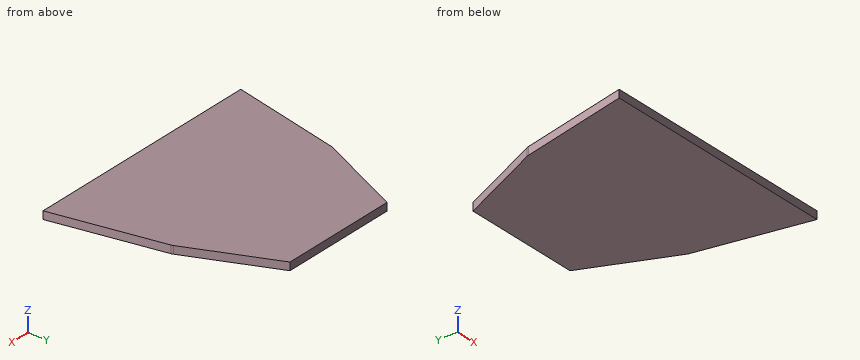
Autodesk Inventor part; units mm, degrees
ref_plane "Work Plane1" through (16.5341, 952.9567, 0) normal (0, 0, 1) x (-1, 0, 0)
ref_plane "YZ Plane" through (0, 0, 0) normal (1, 0, 0) x (0, 1, 0)
ref_plane "XZ Plane" through (0, 0, 0) normal (0, 1, 0) x (-1, 0, 0)
ref_plane "Work Plane1" through (16.5341, 952.9567, 0) normal (0, 0, 1) x (-1, 0, 0)
sketch "Sketch1" plane through (16.5341, 952.9567, 0) normal (0, 0, 1) x (-1, 0, 0)
  line L0 (60, 40.2719) -> (60, 137.1193)
  ellipse E0 centre (56, 137.1193) end of major axis (56, 141.9614) minor radius 4 (60, 137.1193) -> (56, 141.9614) ccw
  line L1 (56, 141.9614) -> (24.75, 141.9614)
  line L2 (24.75, 141.9614) -> (24.75, 144.3824)
  line L3 (24.75, 144.3824) -> (24.75, 146.8034)
  line L4 (24.75, 146.8034) -> (56, 146.8034)
  ellipse E1 centre (56, 137.1193) end of major axis (56, 146.8034) minor radius 8 (64, 137.1193) -> (56, 146.8034) ccw
  line L5 (64, 137.1193) -> (64, 40.2719)
  ellipse E2 centre (56, 40.2719) end of major axis (56, 30.5879) minor radius 8 (63.7591, 37.9134) -> (64, 40.2719) ccw
  line L6 (63.7591, 37.9134) -> (43.4204, -60.1335)
  ellipse E3 centre (35.6613, -57.775) end of major axis (35.6613, -67.459) minor radius 8 (42.7123, -62.3499) -> (43.4204, -60.1335) ccw
  line L7 (42.7123, -62.3499) -> (7.051, -142.8866)
  ellipse E4 centre (0, -138.3116) end of major axis (0, -147.9957) minor radius 8 (-7.051, -142.8866) -> (7.051, -142.8866) ccw
  line L8 (-7.051, -142.8866) -> (-42.7123, -62.3499)
  ellipse E5 centre (-35.6613, -57.775) end of major axis (-35.6613, -67.459) minor radius 8 (-43.4204, -60.1335) -> (-42.7123, -62.3499) ccw
  line L9 (-43.4204, -60.1335) -> (-63.7591, 37.9134)
  ellipse E6 centre (-56, 40.2719) end of major axis (-56, 30.5879) minor radius 8 (-64, 40.2719) -> (-63.7591, 37.9134) ccw
  line L10 (-64, 40.2719) -> (-64, 137.1193)
  ellipse E7 centre (-56, 137.1193) end of major axis (-56, 146.8034) minor radius 8 (-56, 146.8034) -> (-64, 137.1193) ccw
  line L11 (-56, 146.8034) -> (-24.75, 146.8034)
  line L12 (-24.75, 146.8034) -> (-24.75, 144.3824)
  line L13 (-24.75, 144.3824) -> (-24.75, 141.9614)
  line L14 (-24.75, 141.9614) -> (-56, 141.9614)
  ellipse E8 centre (-56, 137.1193) end of major axis (-56, 141.9614) minor radius 4 (-56, 141.9614) -> (-60, 137.1193) ccw
  line L15 (-60, 137.1193) -> (-60, 40.2719)
  ellipse E9 centre (-56, 40.2719) end of major axis (-56, 35.4299) minor radius 4 (-60, 40.2719) -> (-59.8796, 39.0927) ccw
  line L16 (-59.8796, 39.0927) -> (-39.5409, -58.9542)
  ellipse E10 centre (-35.6613, -57.775) end of major axis (-35.6613, -62.617) minor radius 4 (-39.5409, -58.9542) -> (-39.1868, -60.0624) ccw
  line L17 (-39.1868, -60.0624) -> (-3.5255, -140.5991)
  ellipse E11 centre (0, -138.3116) end of major axis (0, -143.1536) minor radius 4 (-3.5255, -140.5991) -> (3.5255, -140.5991) ccw
  line L18 (3.5255, -140.5991) -> (39.1868, -60.0624)
  ellipse E12 centre (35.6613, -57.775) end of major axis (35.6613, -62.617) minor radius 4 (39.1868, -60.0624) -> (39.5409, -58.9542) ccw
  line L19 (39.5409, -58.9542) -> (59.8796, 39.0927)
  ellipse E13 centre (56, 40.2719) end of major axis (56, 35.4299) minor radius 4 (59.8796, 39.0927) -> (60, 40.2719) ccw
  line L20 (-24.75, 141.9614) -> (24.75, 141.9614)
  line L21 (-24.0389, -94.2722) -> (24.0389, -94.2722)
  line L22 (-48.8096, -14.2722) -> (48.8096, -14.2722)
  point P0 (16.5341, 952.9567)
  point P1 (60, -19.5271)
  dimension "d3" = 88.0788
  dimension "d4" = 44.0394
  dimension "d12" = 80
extrude "Plate1" add sketch "Sketch1" along normal blind 3 contours L19 E12 L18 L21 L17 E10 L16 L22
ref_plane "modplan parallel med plade" through (16.5341, 952.9567, 1.5) normal (0, 0, 1) x (1, 0, 0)
sketch "Sketch3" plane through (16.5341, 952.9567, 0) normal (0, 0, -1) x (-1, 0, 0)
  ellipse E0 centre (-35.6613, 57.775) end of major axis (-35.6613, 62.617) minor radius 4 (-39.1868, 60.0624) -> (-39.5409, 58.9542) ccw
  line L0 (-48.8096, 14.2722) -> (-39.5409, 58.9542)
  line L1 (48.8096, 14.2722) -> (-48.8096, 14.2722)
  line L2 (39.5409, 58.9542) -> (48.8096, 14.2722)
  ellipse E1 centre (35.6613, 57.775) end of major axis (35.6613, 62.617) minor radius 4 (39.5409, 58.9542) -> (39.1868, 60.0624) ccw
  line L3 (24.0389, 94.2722) -> (39.1868, 60.0624)
  line L4 (-24.0389, 94.2722) -> (24.0389, 94.2722)
  line L5 (-39.1868, 60.0624) -> (-24.0389, 94.2722)
  line L6 (-37.3581, 59.2527) -> (-22.7372, 92.2722)
  line L7 (-22.7372, 92.2722) -> (22.7372, 92.2722)
  line L8 (22.7372, 92.2722) -> (37.3581, 59.2527)
  line L9 (37.5826, 58.548) -> (46.3522, 16.2722)
  line L10 (46.3522, 16.2722) -> (-46.3522, 16.2722)
  line L11 (-46.3522, 16.2722) -> (-37.5826, 58.548)
  spline S0 degree 3 poles (-37.5826, 58.548) (-37.5324, 58.7898) (-37.4581, 59.0268) (-37.3581, 59.2527) knots 0 0 0 0 1 1 1 1
  spline S1 degree 3 poles (37.3581, 59.2527) (37.4581, 59.0268) (37.5324, 58.7898) (37.5826, 58.548) knots 0 0 0 0 1 1 1 1
  point P0 (16.5341, -952.9567)
  dimension "d14" = 2
extrude "2 mm mindre" cut sketch "Sketch3" against normal blind 3
ref_plane "midtplan" through (16.5341, 1192.6796, 0) normal (-1, 0, 0) x (0, 0, 1)
equation "\"d15\" = Thickness"
equation "\"d8\" = Thickness"
equation "\"Thickness\" = pladetykkelse"
equation "\"BendRadius\" = Thickness"
equation "\"BendReliefWidth\" = Thickness"
equation "\"BendReliefDepth\" = 0.5 * Thickness"
equation "\"CornerReliefSize\" = 4 * Thickness"
equation "\"MinimumRemnant\" = 2 * Thickness"
equation "\"TransitionRadius\" = BendRadius"
equation "\"JacobiRadiusSize\" = BendRadius"
equation "\"GapSize\" = Thickness"
equation "\"pladetykkelse\" = 3"
equation "\"trappevinkel\" = 34.3deg"
equation "\"trappestifter_dia\" = 25"
equation "\"trappestifter_huldia\" = 25.8"
equation "\"trappestifter_skraa_huldia\" = 26.6"
equation "\"trappestifter_laengde\" = 228"
equation "\"perforeringsbredde\" = 6"
equation "\"perforeringshullaengde\" = 62.8"
equation "\"perforeringshullaengde_top\" = 61"
equation "\"perforeringshullaengde_bund\" = 61.6"
equation "\"perforeringsoffset\" = 8"
equation "\"perforeringsoffset_top\" = 8"
equation "\"perforeringsoffset_bund\" = 8"
equation "\"laskehul_dia\" = 13"
equation "\"balusterhul_udvidelse\" = 1"
equation "\"trinbredde\" = 1884"
properties part number "skot" material "S355MC"
The listing builds one solid part. Answer for the finished solid, in the listing's coordinates (mm). Give positions to 0.01 mm unless a question says otherwise; leave off trailing zeros. Order: outer loops, then holes, each group sorted by start corner. A loop starts at its lowest first (then second) coordinate and runs counter-clockwise, first axis right, second up. Notation, with made-up numbers: (25, -23.5) - (79, -23.5) arc R13 cw to (79, -7.5) - close; hole circle Ø8 at (-39, 19.5). An arc over 180 degrees is marked (long way). One line per item, written item: value. Start each with the question number.
1) Given pin 1 Ø1.5 at (y, z) = (1029.5, 0.5) entering from -X; pin 2 Ø1.5 at (y, z) = (1008.5, 2.5) entering from -X, each flat-ended and moving along its own axis, determine where each tip first touches the part or whether it passes through.
2) A cutting plane is placed at A-A on y = 982.5. Give the vertices of the cut face in (x, z), then the cut area to 3 significant figures.
3) Find the intervals of material crossed by L1, parallel to X at y = 1011, z = 1.45; L2, parallel to X at y = 990.5, z = 0.65; L3, parallel to Y at x = -15.5, z = 1.6, in increasing order.
4) A cutting plane is placed at B-B on x = -14. Give the vertices of the cut face in (y, z), then the cut area to 3 significant figures.
Answer sheet:
1. pin 1: stops at x = -13.5
1. pin 2: stops at x = -21.83
2. outline: (-27.07, 0) - (60.13, 0) - (60.13, 3) - (-27.07, 3) - close
2. area: 262 mm2
3. L1: x = -21.15 to 54.22
3. L2: x = -25.41 to 58.47
3. L3: y = 969.23 to 1024.23
4. outline: (969.23, 0) - (1027.62, 0) - (1027.62, 3) - (969.23, 3) - close
4. area: 175 mm2
